from build123d import *

# Parameters (mm, degrees)
SKETCH_1_W          = 221.2
SKETCH_1_H          = 217.66
SKETCH_1_R          = 2.757404821
EXTRUDE_1_DEPTH     = 3
SKETCH_2_R          = 2.55
CUT_EXTRUDE_1_DEPTH = 10
CUT_EXTRUDE_2_DEPTH = 10
FILLET_1_R          = 10
CUT_EXTRUDE_3_DEPTH = 10
FILLET_2_R          = 5


with BuildPart() as part:
    # 草图1 → 凸台-拉伸1 (new body)
    with BuildSketch(Plane.XY):
        with Locations((39.694458169, -239.311229018)):
            Rectangle(SKETCH_1_W, SKETCH_1_H)
        with Locations((-49.205541831, -334.072837073)):
            Circle(SKETCH_1_R, mode=Mode.SUBTRACT)
        with Locations((-36.505541831, -334.072837073)):
            Circle(SKETCH_1_R, mode=Mode.SUBTRACT)
        with Locations((-23.805541831, -334.072837073)):
            Circle(SKETCH_1_R, mode=Mode.SUBTRACT)
        with Locations((-11.105541831, -334.072837073)):
            Circle(SKETCH_1_R, mode=Mode.SUBTRACT)
        with Locations((1.594458169, -334.072837073)):
            Circle(SKETCH_1_R, mode=Mode.SUBTRACT)
        with Locations((14.294458169, -334.072837073)):
            Circle(SKETCH_1_R, mode=Mode.SUBTRACT)
        with Locations((26.994458169, -334.072837073)):
            Circle(SKETCH_1_R, mode=Mode.SUBTRACT)
        with Locations((39.694458169, -334.072837073)):
            Circle(SKETCH_1_R, mode=Mode.SUBTRACT)
        with Locations((52.394458169, -334.072837073)):
            Circle(SKETCH_1_R, mode=Mode.SUBTRACT)
        with Locations((65.094458169, -334.072837073)):
            Circle(SKETCH_1_R, mode=Mode.SUBTRACT)
        with Locations((77.794458169, -334.072837073)):
            Circle(SKETCH_1_R, mode=Mode.SUBTRACT)
        with Locations((90.494458169, -334.072837073)):
            Circle(SKETCH_1_R, mode=Mode.SUBTRACT)
        with Locations((103.194458169, -334.072837073)):
            Circle(SKETCH_1_R, mode=Mode.SUBTRACT)
        with Locations((115.894458169, -334.072837073)):
            Circle(SKETCH_1_R, mode=Mode.SUBTRACT)
        with Locations((-61.905541831, -334.072837073)):
            Circle(SKETCH_1_R, mode=Mode.SUBTRACT)
        with Locations((128.594458169, -334.072837073)):
            Circle(SKETCH_1_R, mode=Mode.SUBTRACT)
        with Locations((141.294458169, -334.072837073)):
            Circle(SKETCH_1_R, mode=Mode.SUBTRACT)
    extrude(amount=EXTRUDE_1_DEPTH)

    # 草图2 → 切除-拉伸1 (cut)
    with BuildSketch(Plane.XY.offset(3)):
        with Locations((-55.905541831, -143.181229018)):
            Circle(SKETCH_2_R)
        with Locations((-55.905541831, -155.881229018)):
            Circle(SKETCH_2_R)
        with Locations((-55.905541831, -168.581229018)):
            Circle(SKETCH_2_R)
        with Locations((-55.905541831, -181.281229018)):
            Circle(SKETCH_2_R)
        with Locations((-55.905541831, -193.981229018)):
            Circle(SKETCH_2_R)
        with Locations((-55.905541831, -206.681229018)):
            Circle(SKETCH_2_R)
        with Locations((-55.905541831, -219.381229018)):
            Circle(SKETCH_2_R)
        with Locations((-55.905541831, -232.081229018)):
            Circle(SKETCH_2_R)
        with Locations((-55.905541831, -244.781229018)):
            Circle(SKETCH_2_R)
        with Locations((-55.905541831, -257.481229018)):
            Circle(SKETCH_2_R)
        with Locations((-55.905541831, -270.181229018)):
            Circle(SKETCH_2_R)
        with Locations((-55.905541831, -282.881229018)):
            Circle(SKETCH_2_R)
        with Locations((-55.905541831, -295.581229018)):
            Circle(SKETCH_2_R)
        with Locations((-55.905541831, -308.281229018)):
            Circle(SKETCH_2_R)
        with Locations((-55.905541831, -320.981229018)):
            Circle(SKETCH_2_R)
        with Locations((135.294458169, -320.981229018)):
            Circle(SKETCH_2_R)
        with Locations((135.294458169, -308.281229018)):
            Circle(SKETCH_2_R)
        with Locations((135.294458169, -295.581229018)):
            Circle(SKETCH_2_R)
        with Locations((135.294458169, -282.881229018)):
            Circle(SKETCH_2_R)
        with Locations((135.294458169, -270.181229018)):
            Circle(SKETCH_2_R)
        with Locations((135.294458169, -257.481229018)):
            Circle(SKETCH_2_R)
        with Locations((135.294458169, -244.781229018)):
            Circle(SKETCH_2_R)
        with Locations((135.294458169, -232.081229018)):
            Circle(SKETCH_2_R)
        with Locations((135.294458169, -219.381229018)):
            Circle(SKETCH_2_R)
        with Locations((135.294458169, -206.681229018)):
            Circle(SKETCH_2_R)
        with Locations((135.294458169, -193.981229018)):
            Circle(SKETCH_2_R)
        with Locations((135.294458169, -181.281229018)):
            Circle(SKETCH_2_R)
        with Locations((135.294458169, -168.581229018)):
            Circle(SKETCH_2_R)
        with Locations((135.294458169, -155.881229018)):
            Circle(SKETCH_2_R)
        with Locations((135.294458169, -143.181229018)):
            Circle(SKETCH_2_R)
    extrude(amount=-CUT_EXTRUDE_1_DEPTH, mode=Mode.SUBTRACT)

    # 草图3 → 切除-拉伸2 (cut)
    with BuildSketch(Plane.XY.offset(3)):
        Polygon((112.294458169, -345.141229018), (112.294458169, -328.141229018), (134.294458169, -276.141229018), (150.294458169, -276.141229018), (150.294458169, -348.141229018), (-70.905541831, -348.141229018), (-70.905541831, -276.141229018), (-54.905541831, -276.141229018), (-32.905541831, -328.141229018), (-32.905541831, -345.141229018), align=None)
    extrude(amount=-CUT_EXTRUDE_2_DEPTH, mode=Mode.SUBTRACT)

    # 圆角1
    fillet_1_edges = [part.edges().sort_by_distance(p)[0] for p in [
        (150.294458169, -276.141229018, 1.5),
        (112.294458169, -328.141229018, 1.5),
        (-32.905541831, -328.141229018, 1.5),
        (-32.905541831, -345.141229018, 1.5),
        (112.294458169, -345.141229018, 1.5),
        (-70.905541831, -276.141229018, 1.5),
        (-70.905541831, -130.481229018, 1.5),
        (150.294458169, -130.481229018, 1.5),
    ]]
    fillet(fillet_1_edges, radius=FILLET_1_R)

    # 草图4 → 切除-拉伸3 (cut)
    with BuildSketch(Plane.XY.offset(3)):
        Polygon((-15.305541831, -179.721297416), (27.293741344, -237.811229018), (-15.305541831, -295.90116062), align=None)
        Polygon((-2.904825006, -162.811229018), (82.293741344, -162.811229018), (39.694458169, -220.90116062), align=None)
        Polygon((-2.904825006, -312.811229018), (82.293741344, -312.811229018), (39.694458169, -254.721297416), align=None)
        Polygon((94.694458169, -179.721297416), (94.694458169, -295.90116062), (52.095174994, -237.811229018), align=None)
    extrude(amount=-CUT_EXTRUDE_3_DEPTH, mode=Mode.SUBTRACT)

    # 圆角2
    fillet_2_edges = [part.edges().sort_by_distance(p)[0] for p in [
        (-2.904825006, -312.811229018, 1.5),
        (39.694458169, -254.721297416, 1.5),
        (82.293741344, -312.811229018, 1.5),
        (-15.305541831, -295.90116062, 1.5),
        (-15.305541831, -179.721297416, 1.5),
        (27.293741344, -237.811229018, 1.5),
        (94.694458169, -295.90116062, 1.5),
        (52.095174994, -237.811229018, 1.5),
        (94.694458169, -179.721297416, 1.5),
        (39.694458169, -220.90116062, 1.5),
        (-2.904825006, -162.811229018, 1.5),
        (82.293741344, -162.811229018, 1.5),
    ]]
    fillet(fillet_2_edges, radius=FILLET_2_R)


solid = part.part
Build history of the part. All positions in model axes, mm. A direction names the side the tool comes from. Give positions to 0.01 mm unless a question says otherwise; leave off trailing zeros. Order: outer loops, then holes, each group sorted by start corner. A loop starts at its lowest first (then second) coordinate and runs counter-clockwise, first axis right, second up. Notation, with made-up numbers: M -31,73 L 16,73 A27 ccw 16,102 Z; hole C 48.25,-16.5 d10. An arc over 180 degrees is marked long. Put each result on its own line as item: value.
Item 1: Slice it at D-D, the plane y = -317. Write the cut outline in (x, z), plus the area to 3 significant figures.
From the geometry:
outline: M -37.62,0 L 117.01,0 L 117.01,3 L -37.62,3 Z
area: 464 mm2
Item 2: Slice it at A-A, the plane y = -187. Write the cut outline in (x, z), plus the area to 3 significant figures.
From the geometry:
outline: M -70.91,0 L 14.83,0 L 14.83,3 L -70.91,3 Z; M 64.56,0 L 150.29,0 L 150.29,3 L 64.56,3 Z
area: 514 mm2
Item 3: Two-plate mould, pull along Y, no slides. Class faces 1 (the flat face through (60.3, -192.8, 1.5)), 2 (the cylindrical face through (-68.054, -133.488, 1.521)), 3 (the flat face through (-44.449, -300.856, 1.521)): +Y half, -Y half, draft (parallel to the pull), parting line (faces both ways), or undercut.
From the geometry:
face 1: undercut
face 2: +Y half
face 3: -Y half
Item 4: Probe line 1 (Y direction, x = 60, z = 0.9); line 2 (X direction, y = -266, z = 1.25); line 3 (X direction, y = -278, z = 2.4). List the from-to ranges inside material, lowest first. Write a range as [from, to].
From the geometry:
line 1: y = [-345.14, -312.81], [-282.41, -248.59], [-227.03, -193.21], [-162.81, -130.48]
line 2: x = [-70.91, -15.31], [6.62, 31.42], [47.97, 72.77], [94.69, 150.29]
line 3: x = [-54.12, -15.31], [-2.18, 22.62], [56.77, 81.57], [94.69, 133.51]
Item 5: Slice it at C-C, the plane z = 1.2. Give the number of separate pieces and of enclosed holes in the cut face, plus the area to 3 significant figures.
From the geometry:
separate pieces: 1
enclosed holes: 37
area: 32,900 mm2
Item 6: 3-axis set-ups, long thin cutter, end or side, ignore diameter. For faces 4 (the flat face through (69.74, -213.75, 1.52)), 5 (the flat face through (38, -236, 0)): which of +Z, -Z, +X, -X, +Y, -Y reach the whole face in a straight line?
From the geometry:
face 4: +Z, -Z
face 5: -Z, +X, -X, +Y, -Y
Item 7: Flat gauge pins, fed straight in: pin 1 Ø4.5 at (x, y) = (26.99, -334.07) entering from -Z; pin 2 Ø10 at (x, y) = (44.5, -312.5) entering from -Z. Where does each tip first touch, or does it go through?
From the geometry:
pin 1: passes through
pin 2: stops at z = 0
Item 8: Slice it at B-B, the plane x = 58. Write the cut outline in (y, z).
From the geometry:
outline: M -345.14,0 L -312.81,0 L -312.81,3 L -345.14,3 Z; M -279.68,0 L -245.86,0 L -245.86,3 L -279.68,3 Z; M -229.76,0 L -195.94,0 L -195.94,3 L -229.76,3 Z; M -162.81,0 L -130.48,0 L -130.48,3 L -162.81,3 Z
